from build123d import *

# Parameters (mm, degrees)
SKETCH1_W            = 501.65
SKETCH1_H            = 88.9
BOSS_EXTRUDE1_DEPTH  = 309.5625
SKETCH2_W            = 349.25
SKETCH2_H            = 7.9375
CUT_EXTRUDE1_DEPTH   = 401.896401245
FILLET1_R            = 25.4
CUT_EXTRUDE2_DEPTH   = 119.85625
FILLET2_R            = 19.05
CUT_EXTRUDE4_DEPTH   = 41.275
SKETCH4_W            = 396.875
SKETCH4_H            = 284.1625
CUT_EXTRUDE3_DEPTH   = 61.9125
SKETCH6_W            = 82.55
SKETCH6_H            = 39.6875
CUT_EXTRUDE5_DEPTH   = 33.3375
FILLET3_R            = 6.35
SKETCH7_R            = 6.35
CUT_EXTRUDE6_DEPTH   = 401.896401245
FILLET3_OF_MIRROR5_R = 6.35


# Some blends are built 0.0001 mm under size
with BuildPart() as part:
    # Sketch1 → Boss-Extrude1 (new body)
    with BuildSketch(Plane.XY):
        Rectangle(SKETCH1_W, SKETCH1_H)
    extrude(amount=BOSS_EXTRUDE1_DEPTH)

    # Sketch2 → Cut-Extrude1 (cut, through all)
    with BuildSketch(Plane.XY.offset(309.5625)):
        with Locations((0, -40.48125)):
            Rectangle(SKETCH2_W, SKETCH2_H)
    extrude(amount=-CUT_EXTRUDE1_DEPTH, mode=Mode.SUBTRACT)

    # Fillet1
    # the kernel refuses this fillet: 25.4 mm, written as the material it adds along each edge
    with BuildSketch(Plane(origin=(174.625, -36.5125, 309.5625), x_dir=(0, -1, 0), z_dir=(0, 0, -1))) as fillet1_piece_1:
        with BuildLine():
            CenterArc((25.4, 18.445083186), FILLET1_R, 180, 46.567463442)
            Line((0, 18.445083186), (-0.508, 18.445083186))
            Line((-0.508, 18.445083186), (-0.508, 0))
            Line((-0.508, 0), (0, -0.508))
            ThreePointArc((0, -0.508), (3.96875, -0.508), (7.58825, -0.368901664))
            Line((7.58825, -0.368901664), (7.9375, 0))
        make_face()
    extrude(amount=309.5625)
    with BuildSketch(Plane(origin=(-174.625, -36.5125, 309.5625), x_dir=(0, -1, 0), z_dir=(0, 0, -1))) as fillet1_piece_2:
        with BuildLine():
            CenterArc((25.4, -18.445083186), FILLET1_R, 133.432536558, 46.567463442)
            Line((0, -18.445083186), (-0.508, -18.445083186))
            Line((-0.508, -18.445083186), (-0.508, 0))
            Line((-0.508, 0), (0, 0.508))
            ThreePointArc((0, 0.508), (3.96875, 0.508), (7.58825, 0.368901664))
            Line((7.58825, 0.368901664), (7.9375, 0))
        make_face()
    extrude(amount=309.5625)

    # Sketch3 → Cut-Extrude2 (cut, symmetric)
    with BuildSketch(Plane.XY.offset(154.78125)):
        Polygon((-250.825, 44.45), (-233.3625, 44.45), (-250.825, 10.5874677), align=None)
    cut_extrude2 = extrude(amount=CUT_EXTRUDE2_DEPTH, both=True, mode=Mode.SUBTRACT)

    # Fillet2
    fillet2_edges = [part.edges().sort_by_distance(p)[0] for p in [
        (250.825, 44.45, 154.78125),
    ]]
    fillet(fillet2_edges, radius=FILLET2_R)
    # the kernel refuses this fillet: 19.05 mm, written as the material it takes off along each edge
    with BuildSketch(Plane(origin=(-250.825, 44.45, -47.625), x_dir=(1, 0, 0), z_dir=(0, 0, 1))) as fillet2_2_piece_1:
        with BuildLine():
            CenterArc((FILLET2_R, -FILLET2_R), FILLET2_R, 90, 90)
            Line((0, -FILLET2_R), (-FILLET2_R * 0.02, -FILLET2_R))
            Line((-FILLET2_R * 0.02, -FILLET2_R), (-FILLET2_R * 0.02, FILLET2_R * 0.02))
            Line((-FILLET2_R * 0.02, FILLET2_R * 0.02), (FILLET2_R, FILLET2_R * 0.02))
            Line((FILLET2_R, FILLET2_R * 0.02), (FILLET2_R, 0))
        make_face()
    extrude(amount=130.175, mode=Mode.SUBTRACT)
    fillet2_3_edges = [part.edges().sort_by_distance(p)[0] for p in [
        (-250.825, 44.45, 292.1),
    ]]
    fillet(fillet2_3_edges, radius=FILLET2_R - 0.0001)  # a hair under: the kernel refuses the full size

    # Sketch5 → Cut-Extrude4 (cut)
    with BuildSketch(Plane.ZY.offset(250.825)):
        with BuildLine():
            Line((135.73125, 0), (173.83125, 0))
            ThreePointArc((173.83125, 0), (188.11875, -14.2875), (173.83125, -28.575))
            Line((173.83125, -28.575), (135.73125, -28.575))
            ThreePointArc((135.73125, -28.575), (121.44375, -14.2875), (135.73125, 0))
        make_face()
    cut_extrude4 = extrude(amount=-CUT_EXTRUDE4_DEPTH, mode=Mode.SUBTRACT)

    # Mirror4: Cut-Extrude2, Cut-Extrude4 across plane
    add(cut_extrude2.mirror(Plane.ZY), mode=Mode.SUBTRACT)
    add(cut_extrude4.mirror(Plane.ZY), mode=Mode.SUBTRACT)

    # Sketch4 → Cut-Extrude3 (cut)
    with BuildSketch(Plane(origin=(0, 44.45, 0), x_dir=(1, 0, 0), z_dir=(0, 1, 0))):
        with Locations((0, -154.78125)):
            Rectangle(SKETCH4_W, SKETCH4_H)
    extrude(amount=-CUT_EXTRUDE3_DEPTH, mode=Mode.SUBTRACT)

    # Sketch6 → Cut-Extrude5 (cut)
    with BuildSketch(Plane.ZY.offset(198.4375)):
        with Locations((154.78125, 2.38125)):
            Rectangle(SKETCH6_W, SKETCH6_H)
    cut_extrude5 = extrude(amount=CUT_EXTRUDE5_DEPTH, mode=Mode.SUBTRACT)

    # Fillet3
    fillet3_edges = [part.edges().sort_by_distance(p)[0] for p in [
        (-215.10625, 22.225, 196.05625),
        (-215.10625, 22.225, 113.50625),
    ]]
    fillet(fillet3_edges, radius=FILLET3_R)

    # Sketch7 → Cut-Extrude6 (cut, through all)
    with BuildSketch(Plane.XY.offset(309.5625)):
        with Locations((-47.625, 28.575)):
            Circle(SKETCH7_R)
        with Locations((-142.875, 28.575)):
            Circle(SKETCH7_R)
    cut_extrude6 = extrude(amount=-CUT_EXTRUDE6_DEPTH, mode=Mode.SUBTRACT)

    # Mirror5: Cut-Extrude5, Cut-Extrude6 across plane
    add(cut_extrude5.mirror(Plane.ZY), mode=Mode.SUBTRACT)
    add(cut_extrude6.mirror(Plane.ZY), mode=Mode.SUBTRACT)

    # Fillet3 of Mirror5
    fillet3_of_mirror5_edges = [part.edges().sort_by_distance(p)[0] for p in [
        (215.10625, 22.225, 196.05625),
        (215.10625, 22.225, 113.50625),
    ]]
    fillet(fillet3_of_mirror5_edges, radius=FILLET3_OF_MIRROR5_R)


solid = part.part
Check sheet for the modelled part. Datum: model origin and axes. Units: mm. A direction names the side the tool comes from. Round coordinates to 2 decimals unless told otherwise and drop trailing zeros. Write each loop counter-clockwise with the first axis right and the second up, starting at its lowest first coordinate (ties: lowest second). Pieces come first, ordered by that corner, then holes. Notation, with made-up numbers: (-3.5, -5.5) - (17.5, -5.5) arc R14 ccw to (17.5, 12.5) - close; hole circle Ø4 at (34, 54). An arc over 180 degrees is marked (long way). Return JSON: item names as keys, results as strings.
Q1. Draft check along X on faces 1 (the flat face through (-209.55, -23, 155)), 2 (the cylindrical face through (-235.06, -18.88, 187.36)), 3 (the flat face through (250.825, -33, 153)), 4 (the cylindrical face through (-137.01, 26.14, 6.44)). Enter one of: released by +X, released by -X, zero draft, split by the parting line, or undercut.
Returned:
{"face 1": "released by -X", "face 2": "zero draft", "face 3": "released by +X", "face 4": "undercut"}
Q2. Cross-section at A-A (z = 151). Give the number of separate pieces and of enclosed holes in the cut face, then the cut area to 3 significant figures.
Returned:
{"separate pieces": "3", "enclosed holes": "0", "area": "12,500 mm²"}
Q3. Depth check by flat-ended pin: P1, Ø1, axis at x = -84, z = 175.5, coming from the -Y side; P2, Ø11.5, axis at x = 142.875, y = 28.575, coming from the +Z side; P3, Ø3, axis at x = -193.5, z = 199, coming from the +Y side; P4, Ø3.5, axis at y = -20.5, z = 160, coming from the -X side. Enter the tip coordinate at first touch or a pass-through.
Returned:
{"P1": "stops at y = -36.51", "P2": "passes through", "P3": "stops at y = -17.46", "P4": "stops at x = -209.55"}
Q4. Access from +Z, -Z, +X, -X, +Y, -Y to the whole of each face (thin tool, end or side, straight path). Record for faces 5 (the flat face through (-244, 31, 274.638)), 6 (the flat face through (-2, -36.512, 157)), 7 (the flat face through (241, 0, 155)), 8 (the flat face through (-215, -1, 196.056)), 9 (the flat face through (-230, -28.575, 155)).
Returned:
{"face 5": "-X, +Y", "face 6": "+Z, -Z, -Y", "face 7": "+X, -X", "face 8": "none", "face 9": "-X"}
Q5. Cross-section at B-B (x = -69.5). Record the boundary of the cut face in (y, z).
Returned:
{"outline": "(-36.51, 0) - (44.45, 0) - (44.45, 12.7) - (-17.46, 12.7) - (-17.46, 296.86) - (44.45, 296.86) - (44.45, 309.56) - (-36.51, 309.56) - close"}
Q6. Scan lines: L1, parallel to X at y = -12, z = 34 (1 decimal); L2, parallel to Z at x = 181.5, y = 24.5; L3, parallel to Y at x = -94.5, z = 248. Record each from-to range of solid material in increasing order. Write a range as from..to.
Returned:
{"L1": "x = -250.8..-198.4, 198.4..250.8", "L2": "z = 0..12.7, 296.86..309.56", "L3": "y = -36.51..-17.46"}
Q7. Cross-section at D-D (y = -10). Record the boundary of the cut face in (x, z) (1 decimal), then the cut area to 3 significant figures.
Returned:
{"outline": "(-250.8, 0) - (250.8, 0) - (250.8, 122.1) - (231.8, 122.1) - (231.8, 113.5) - (198.4, 113.5) - (198.4, 12.7) - (-198.4, 12.7) - (-198.4, 113.5) - (-231.8, 113.5) - (-231.8, 122.1) - (-250.8, 122.1) - close; (-250.8, 187.5) - (-231.8, 187.5) - (-231.8, 196.1) - (-198.4, 196.1) - (-198.4, 296.9) - (198.4, 296.9) - (198.4, 196.1) - (231.8, 196.1) - (231.8, 187.5) - (250.8, 187.5) - (250.8, 309.6) - (-250.8, 309.6) - close", "area": "34,500 mm²"}
